Check sheet for the modelled part. Datum: model origin and axes. Units: mm. Round coordinates to 2 decimals unless told otherwise and drop trailing zeros. Write each loop counter-clockwise with the first axis right and the second up, starting at its lowest first coordinate (ties: lowest second). Pieces come first, ordered by that corner, then holes. Notation, with made-up numbers: (79.25, 39.5) -> (97.25, 39.5) arc R21 ccw to (97.25, 53.5) -> close; hole circle Ø9 at (1, 8). An arc over 180 degrees is marked (long way). Put each result on its own line as item: value. Start each with the question number.
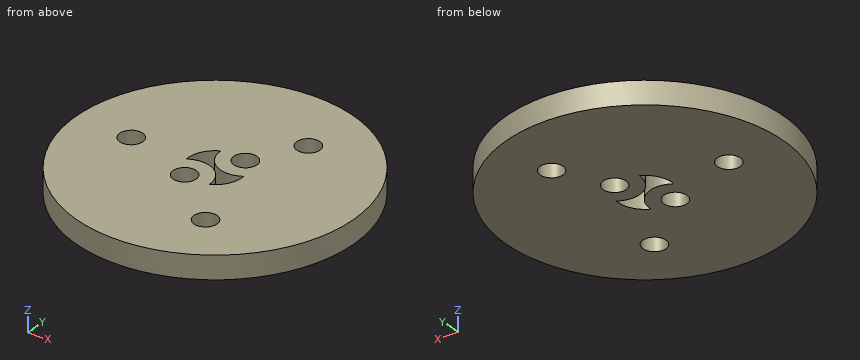
from build123d import *

# Parameters (mm, degrees)
ESQUISSE1_R        = 18
ESQUISSE1_R_2      = 1.5
BOSS_EXTRU_1_DEPTH = 3


with BuildPart() as part:
    # Esquisse1 → Boss.-Extru.1 (new body)
    with BuildSketch(Plane.XY):
        Circle(ESQUISSE1_R)
        with Locations((5.240453276, 9.386167986)):
            Circle(ESQUISSE1_R_2, mode=Mode.SUBTRACT)
        with Locations((-1.70619409, -3.05596167)):
            Circle(ESQUISSE1_R_2, mode=Mode.SUBTRACT)
        with Locations((1.70619409, 3.05596167)):
            Circle(ESQUISSE1_R_2, mode=Mode.SUBTRACT)
        with Locations((5.508433282, -9.231449657)):
            Circle(ESQUISSE1_R_2, mode=Mode.SUBTRACT)
        with Locations((-10.748886558, -0.154718329)):
            Circle(ESQUISSE1_R_2, mode=Mode.SUBTRACT)
        with BuildLine():
            ThreePointArc((1.54267531, -3.141679947), (-0.121871006, -0.218282976), (-3.483906341, -0.335256035))
            ThreePointArc((-3.483906341, -0.335256035), (-3.05596167, 1.70619409), (-1.54267531, 3.141679947))
            ThreePointArc((-1.54267531, 3.141679947), (0.121871006, 0.218282976), (3.483906341, 0.335256035))
            ThreePointArc((3.483906341, 0.335256035), (3.05596167, -1.70619409), (1.54267531, -3.141679947))
        make_face(mode=Mode.SUBTRACT)
    extrude(amount=BOSS_EXTRU_1_DEPTH)


solid = part.part
1. Section check C-C, the plane z = 2.1. Enter the section's corners in (x, y).
2. Gauge pin test, flat ends, axial feed: P1, Ø1.8, axis at x = 1.71, y = 3.06, coming from the +Z side; P2, Ø1, axis at x = -1.5, y = -8, coming from the -Z side; P3, Ø1.5, axis at x = 8.5, z = 1, coming from the +Y side. Record the tip position at first contact, or that the pin passes through.
3. Section check B-B, the plane x = 2. Enter the section's corners in (y, z), then the cut area to 3 significant figures.
4. Material ranges on L1, parallel to Y at x = -0.5, z = 1.3; L2, parallel to X at y = -3, z = 1; L3, parallel to Y at x = 6, z = 1.1, recorded low to high. Write a range as [from, to].
5. Section check D-D, the plane x = -7. Enter the section's corners in (y, z).
6. Section check A-A, the plane y = -10. Enter the section's corners in (x, z), then the cut area to 3 significant figures.
Reply:
1. outline: circle Ø36 at (0, 0); hole circle Ø3 at (-10.75, -0.15); hole (-3.48, -0.34) arc R3.25 cw to (1.54, -3.14) arc R3.5 ccw to (3.48, 0.34) arc R3.25 cw to (-1.54, 3.14) arc R3.5 ccw to start; hole circle Ø3 at (-1.71, -3.06); hole circle Ø3 at (1.71, 3.06); hole circle Ø3 at (5.24, 9.39); hole circle Ø3 at (5.51, -9.23)
2. P1: passes through
2. P2: stops at z = 0
2. P3: stops at y = 16.25
3. outline: (-17.89, 0) -> (-2.87, 0) -> (-2.87, 3) -> (-17.89, 3) -> close; (-0.18, 0) -> (1.59, 0) -> (1.59, 3) -> (-0.18, 3) -> close; (4.53, 0) -> (17.89, 0) -> (17.89, 3) -> (4.53, 3) -> close
3. area: 90.4 mm2
4. L1: y = [-17.99, -3.95], [-2.16, -0.04], [0.67, 17.99]
4. L2: x = [-17.75, -3.21], [-0.21, 1.54], [1.8, 17.75]
4. L3: y = [-16.97, -10.65], [-7.81, 8.09], [10.68, 16.97]
5. outline: (-16.58, 0) -> (16.58, 0) -> (16.58, 3) -> (-16.58, 3) -> close
6. outline: (-14.97, 0) -> (4.22, 0) -> (4.22, 3) -> (-14.97, 3) -> close; (6.8, 0) -> (14.97, 0) -> (14.97, 3) -> (6.8, 3) -> close
6. area: 82.1 mm2
